Autodesk Inventor part; units mm, degrees
ref_plane "YZ Plane" through (0, 0, 0) normal (1, 0, 0) x (0, 1, 0)
ref_plane "XZ Plane" through (0, 0, 0) normal (0, 1, 0) x (-1, 0, 0)
ref_plane "XY Plane" through (0, 0, 0) normal (0, 0, 1) x (1, 0, 0)
sketch "Sketch1" plane through (0, 0, 0) normal (0, 1, 0) x (-1, 0, 0)
  line L0 (269.2628, -287.2233) -> (16.4197, -34.3803)
  circle A0 centre (270.2276, -277.5195) radius 3.3782
  line L1 (287.2233, -269.2628) -> (34.3803, -16.4197)
  line L2 (6.35, -37.5671) -> (6.35, -393.6488)
  line L3 (-6.35, -37.5671) -> (-6.35, -393.7)
  line L4 (-90.8271, -393.7) -> (-29.6915, -23.8752)
  line L5 (-101.6, -381) -> (-37.5898, 6.214)
  circle A1 centre (0, -387.35) radius 3.3782
  line L6 (37.5671, 6.35) -> (393.7, 6.35)
  line L7 (37.5671, -6.35) -> (393.6488, -6.35)
  circle A2 centre (387.35, 0) radius 3.3782
  circle A3 centre (-95.25, -387.35) radius 3.3782
  circle A4 centre (277.5195, -270.2276) radius 3.3782
  line L8 (-101.6, -381) -> (-101.6, -393.7)
  line L9 (393.7, 0) -> (393.7, 6.35)
  arc A5 (6.35, -37.5671) -> (16.4197, -34.3803) centre (0, 0) ccw
  arc A6 (34.3803, -16.4197) -> (37.5671, -6.35) centre (0, 0) ccw
  line L10 (38.1, 0) -> (38.1, 12.8556) construction
  arc A7 (37.5671, 6.35) -> (-37.5898, 6.214) centre (0, 0) ccw
  circle A8 centre (0, 0) radius 38.1 construction
  arc A9 (-6.214, 37.5898) -> (-37.5898, 6.214) centre (0, 0) ccw
  arc A10 (-29.6915, -23.8752) -> (-6.35, -37.5671) centre (0, 0) ccw
  line L11 (146.05, 0) -> (146.05, 6.35)
  line L12 (133.35, 0) -> (133.35, 6.35)
  line L13 (273.05, 6.35) -> (273.05, 0)
  line L14 (285.75, 6.35) -> (285.75, 0)
  circle A11 centre (103.1708, -94.1906) radius 3.3782
  circle A12 centre (94.1906, -103.1708) radius 3.3782
  arc A13 (393.6488, -6.35) -> (393.7, 0) centre (0, 0) ccw
  circle A14 centre (279.4, 0) radius 3.3782
  circle A15 centre (139.7, 0) radius 3.3782
  arc A16 (0, -393.7) -> (6.35, -393.6488) centre (0, 0) ccw
  arc A17 (269.2628, -287.2233) -> (287.2233, -269.2628) centre (0, 0) ccw
  circle A18 centre (202.0047, -193.0245) radius 3.3782
  circle A19 centre (193.0245, -202.0047) radius 3.3782
  circle A20 centre (0, -279.4) radius 3.3782
  line L15 (-101.6, -393.7) -> (-90.8271, -393.7)
  line L16 (-6.35, -393.7) -> (0, -393.7)
  circle A21 centre (0, -139.7) radius 3.3782
  circle A22 centre (0, 0) radius 14.2875
  circle A23 centre (-55.2746, -139.7) radius 3.3782
  circle A24 centre (-78.3684, -279.4) radius 3.3782
  line L17 (0, -285.75) -> (-6.35, -285.75)
  line L18 (-6.35, -273.05) -> (0, -273.05)
  circle A25 centre (0, -336.55) radius 3.3782
  circle A26 centre (-87.8158, -336.55) radius 3.3782
  circle A27 centre (241.5985, -234.3065) radius 3.3782
  circle A28 centre (234.3065, -241.5985) radius 3.3782
  circle A29 centre (336.55, 0) radius 3.3782
  dimension "d0" = 12.7
  dimension "d1" = 101.6
  dimension "d2" = 12.7
  dimension "d3" = 12.7
  dimension "d4" = 38.1
  dimension "d5" = 38.1
  dimension "d6" = 38.1
  dimension "d7" = 6.35
  dimension "d8" = 6.35
  dimension "d9" = 6.35
  dimension "d10" = 12.7
  dimension "d11" = 12.7
  dimension "d12" = 95.25
  dimension "d14" = 6.7564
  dimension "d15" = 6.7564
  dimension "d16" = 6.7564
  dimension "d17" = 6.35
  dimension "d18" = 6.7564
  dimension "d19" = 6.35
  dimension "d20" = 6.35
  dimension "d21" = 6.7564
  dimension "d22" = 6.7564
  dimension "d23" = 6.7564
  dimension "d25" = 6.35
  dimension "d26" = 6.7564
  dimension "d28" = 28.575
  dimension "d30" = 6.7564
  dimension "d32" = 6.7564
  dimension "d36" = 38.1
  dimension "d37" = 25.4
  dimension "d38" = 6.35
  dimension "d39" = 139.7
  dimension "d40" = 55.2746
  dimension "d41" = 139.7
  dimension "d42" = 6.35
  dimension "d43" = 6.35
  dimension "d44" = 7.3006
  dimension "d45" = 277.5195
  dimension "d46" = 270.2276
  dimension "d47" = 7.2919
  dimension "d48" = 7.2919
  dimension "d49" = 393.7
  dimension "d50" = 393.7
  dimension "d51" = 6.35
  dimension "d52" = 12.7
  dimension "d53" = 6.7564
  dimension "d54" = 6.35
  dimension "d55" = 6.7564
  dimension "d56" = 6.7564
  dimension "d57" = 393.7
  dimension "d58" = 6.35
  dimension "d60" = 6.7564
  dimension "d61" = 6.35
  dimension "d62" = 6.7564
  dimension "d63" = 6.7564
  dimension "d64" = 6.7564
  dimension "d65" = 6.7564
  dimension "d66" = 50.8
  dimension "d67" = 50.8
  dimension "d68" = 50.8
  dimension "d71" = 7.5438
  dimension "d72" = 7.5438
  dimension "d73" = 7.5438
  dimension "d74" = 7.5438
extrude "Extrusion2" add sketch "Sketch1" along normal blind 6.35
sketch "Sketch6" plane through (0, 6.35, 0) normal (0, 1, 0) x (1, 0, 0)
  line L0 (-16.4197, 34.3803) -> (-269.2628, 287.2233)
  line L1 (-287.2233, 269.2628) -> (-34.3803, 16.4197)
  line L2 (-393.7, -6.35) -> (-37.5671, -6.35)
  line L3 (101.6, 381) -> (101.6, 393.7)
  arc A0 (0, 393.7) -> (-6.35, 393.6488) centre (0, 0) ccw
  line L4 (0, 0) -> (-287.2233, 287.2233) construction
  circle A1 centre (0, 0) radius 14.2875
  line L5 (-37.5671, 6.35) -> (-393.6488, 6.35)
  line L6 (6.35, 37.5671) -> (6.35, 393.7)
  circle A2 centre (-107.7631, 107.7631) radius 3.3782
  circle A3 centre (-143.6841, 143.6841) radius 3.3782
  line L7 (-146.05, 464.3998) -> (-146.05, -90.5947) construction
  circle A4 centre (-203.2, 0) radius 3.3782
  circle A5 centre (-152.4, 0) radius 3.3782
  line L8 (-146.05, -6.35) -> (-146.05, 6.35)
  line L9 (-209.55, 6.35) -> (-209.55, -6.35)
  line L10 (-139.194, 157.1545) -> (-157.1545, 139.194)
  line L11 (-112.2532, 94.2927) -> (-94.2927, 112.2532)
  line L12 (-209.55, 6.35) -> (-157.1545, 139.194)
  line L13 (-112.2532, 94.2927) -> (-146.05, 6.35)
  line L14 (-183.3522, 72.772) -> (-129.1516, 50.3213)
  dimension "d115" = 6.7564
  dimension "d117" = 6.7564
  dimension "d118" = 247.65
  dimension "d122" = 152.4
  dimension "d123" = 203.2
  dimension "d124" = 6.7564
  dimension "d126" = 152.4
  dimension "d127" = 203.2
  dimension "d129" = 6.35
  dimension "d130" = 6.35
  dimension "d131" = 6.35
  dimension "d132" = 6.35
extrude "Extrusion8" cut sketch "Sketch6" against normal blind 25.4 contours A2 | A3 | A4 | A5
sketch "Sketch8" plane through (0, 6.35, 0) normal (0, 1, 0) x (1, 0, 0)
  circle A0 centre (0, 0) radius 14.2875
  arc A1 (0, 393.7) -> (-6.35, 393.6488) centre (0, 0) ccw
  circle A2 centre (0, 0) radius 9.5
  dimension "d135" = 19
extrude "Extrusion9" add sketch "Sketch8" against normal blind 6.35
sketch "Sketch9" plane through (0, 6.35, 0) normal (0, 1, 0) x (1, 0, 0)
  circle A0 centre (95.25, 365.2157) radius 3.3782
  circle A1 centre (15.875, -28.575) radius 2.54
extrude "Extrusion10" cut sketch "Sketch9" against normal through all
equation "\"d71\" = d74"
equation "\"d72\" = d73"
properties part number "Bearing Mount v1" material "Aluminum 6061"
Can you work these out from the model? Positions are in its coordinate system, mm. A direction names the side the tool comes from. Round coordinates to 2 decimals unless told otherwise and drop trailing zeros. Order: outer loops, then holes, each group sorted by start corner. A loop starts at its lowest first (then second) coordinate and runs counter-clockwise, first axis right, second up. Notation, with made-up numbers: (-37.5, -36.5) -> (21.5, -36.5) arc R12 cw to (21.5, -23.5) -> close; hole circle Ø11 at (79.5, 60.25). An arc over 180 degrees is marked (long way). Return JSON: item names as keys, results as strings. Group by question number.
1. If we section it at A-A, the plane z = -65: Write out the boundary of the cut face in (x, y).
2. We'd pull the mould along X, two halves only. Please class faces 4 (the face through (4.38, 3.22, 8.43)), 5 (the face through (-92, 6.35, -99)), 6 (the face through (19.11, 3.13, -32.96)), 7 (the face through (0.82, 3.13, 38.09)): released by +X, released by -X, zero draft, split by the parting line, or undercut.
3. If we section it at B-B, the plane x = -43.5: Write out the boundary of the cut face in (y, z).
4. Which directions (+Z, -Z, +X, -X, +Y, -Y) give clear straight access to the entire face, cutting with the end or side of a thin tool? Please do faces 1 (the face through (-278.514, 3.131, -278.262)), 2 (the face through (-144.61, 3.13, -162.57)), 3 (the face through (-162.57, 3.13, -144.61)).
5. Will these pins go through, and if not, where does the flat tip stop? pin 1 (6 mm diameter, centred on x = 55.27, z = -139.7, fed in from +Y); pin 2 (3 mm diameter, centred on x = -112.5, y = 1, fed in from -Z); pin 3 (1 mm diameter, centred on y = 5, z = -310, fed in from +X); pin 4 (3 mm diameter, centred on y = 5, z = -317, fed in from +X).
6. If we section it at C-C, the plane y = 4: Count the separate pieces of the cut face and the enclosed holes in it, then the cut area to 3 significant figures.
7. I need wall thicknesses on line 1 (Z direction, x = 0, y = 4.5); line 2 (X direction, y = 3.5, z = -192.5); line 3 (X direction, y = 1, z = -253). Which ranges of each line are inside material? Lowest first, please. Write a range as [from, to].
Output values:
{
 "1": {"outline": "(-82.96, 0) -> (-47.04, 0) -> (-47.04, 6.35) -> (-82.96, 6.35) -> close; (-6.35, 0) -> (6.35, 0) -> (6.35, 6.35) -> (-6.35, 6.35) -> close; (36.49, 0) -> (49.36, 0) -> (49.36, 6.35) -> (36.49, 6.35) -> close"},
 "2": {"face 4": "undercut", "face 5": "zero draft", "face 6": "undercut", "face 7": "split by the parting line"},
 "3": {"outline": "(0, -61.46) -> (6.35, -61.46) -> (6.35, -25.54) -> (0, -25.54) -> close; (0, -6.35) -> (6.35, -6.35) -> (6.35, 6.35) -> (0, 6.35) -> close"},
 "4": {"face 1": "-Z, -X, +Y, -Y", "face 2": "-Z, +Y, -Y", "face 3": "-X, +Y, -Y"},
 "5": {"pin 1": "through", "pin 2": "z = -131.96", "pin 3": "x = 89.95", "pin 4": "x = 91.27"},
 "6": {"separate pieces": "1", "enclosed holes": "27", "area": "26,300 mm²"},
 "7": {"line 1": "[-393.7, -390.73], [-383.97, -339.93], [-333.17, -282.78], [-276.02, -143.08], [-136.32, -9.5], [9.5, 38.1]", "line 2": "[-210.46, -205.34], [-198.67, -174.54], [-6.35, 6.35], [57.57, 70.44]", "line 3": "[-270.96, -235.04], [-6.35, 6.35], [67.57, 80.44]"}
}
